Model file for the job. Use its own axes, mm. Face numbers are marked on the shaded views. Give positions to 0.01 mm unless a question says otherwise; leave off trailing zeros. Loops run counter-clockwise (first coordinate to the right, second up) from the corner with the lowest first, then second, coordinate; pieces in that order, holes last. Notation, with made-up numbers: M -13.5,42.5 L 28.5,42.5 A36 ccw 28.5,80.5 Z; hole C 47,-6 d10. An arc over 180 degrees is marked long. Use CSV: the item, a comma, the result in double quotes. Start each with the question number.
(1) Slice it at C-C on x = -41. List the corners of the cut face in (y, z).
(2) Wall check: line 1 along X through (y, z) = (-11, 9); line 2 along X through (y, z) = (10.75, 2.5); line 3 along Y through (x, z) = (-14.5, 2.25). Give the ranges that are in metal, low to high. Write a range as from..to.
(3) Slice it at B-B on y = -5. List the corners of the cut face in (x, z).
(4) Two-plate mould, pull along X, no slides. Class the marked faces 1, 2 and 3: pulls with the +X half, pulls with the -X half, needs draft (parallel to the pull), parting line crosses it, or undercut.
(5) Flat gauge pins, fed straight in: P1, Ø6, axis at x = 19, z = 18.5, coming from the +Y side; P2, Ø5, axis at x = 8.5, z = 11, coming from the +Y side; P3, Ø4, axis at x = 1.5, z = 15.5, coming from the +Y side. Where does each tip first touch, or does it go through?
(6) Slice it at A-A on x = 9. List the corners of the cut face in (y, z), and give its area (3 significant figures).
```python
from build123d import *

# Parameters (mm, degrees)
F0_W     = 101.6
F0_H     = 25.4
F1_DEPTH = 25.4
F3_DEPTH = 101.6
F4_R     = 2.54
F5_R     = 2.667
F6_DEPTH = 4.064
F7_W     = 22.86
F7_H     = 20.81151
F8_DEPTH = 2.54


with BuildPart() as f1:
    # F0 (on Top) → F1 (new body)
    with BuildSketch(Plane.XY):
        with Locations((0, -0.170567)):
            Rectangle(F0_W, F0_H)
    extrude(amount=F1_DEPTH)

    # F2 (on face) → F3 (cut, through all)
    with BuildSketch(Plane(origin=(-50.8, 0, 0), x_dir=(0, -1, 0), z_dir=(-1, 0, 0))):
        Polygon((-12.529433, 25.4), (-12.529433, 8.090758), (-10.742588, 5.36007), (12.870567, 20.81151), (12.870567, 25.4), align=None)
    extrude(amount=-F3_DEPTH, mode=Mode.SUBTRACT)

    # F4
    f4_edges = [f1.edges().sort_by_distance(p)[0] for p in [
        (50.8, 12.529433, 4.045379),
        (50.8, -0.170567, 0),
        (-50.8, -0.170567, 0),
        (-50.8, 12.529433, 4.045379),
        (0, 12.529433, 0),
    ]]
    fillet(f4_edges, radius=F4_R)

    # F5 (on face) → F6 (join)
    with BuildSketch(Plane(origin=(0, 5.676581, 8.675048), x_dir=(1, 0, 0), z_dir=(0, 0.547549, 0.836774))):
        with Locations((-40.64, -3.343786)):
            Circle(F5_R)
    extrude(amount=F6_DEPTH)

    # F7 (on face) → F8 (cut)
    with BuildSketch(Plane.XZ.offset(12.870567)):
        with Locations((6.35, 10.405755)):
            Rectangle(F7_W, F7_H)
    extrude(amount=-F8_DEPTH, mode=Mode.SUBTRACT)


solid = f1.part
```
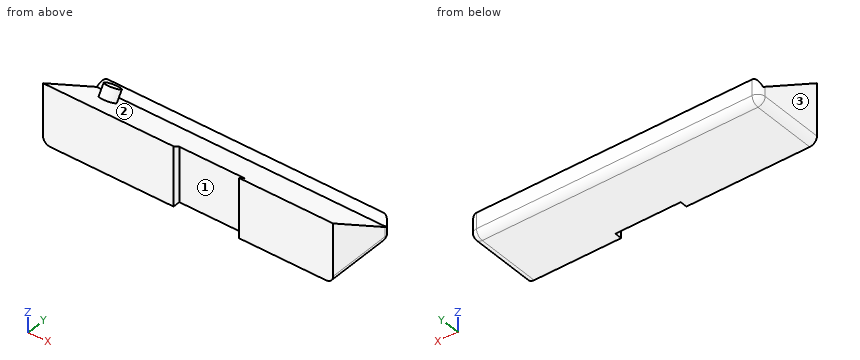
Reply:
1,outline,"M -12.87,0 L 9.99,0 A2.54 ccw 12.53,2.54 L 12.53,8.09 L 10.74,5.36 L 5.09,9.06 L 7.32,12.46 L 2.89,15.35 L 0.67,11.95 L -12.87,20.81 Z"
2,line 1,"x = -50.8..-5.08, 17.78..50.8"
2,line 2,"x = -50.68..50.68"
2,line 3,"y = -12.87..12.51"
3,outline,"M -50.8,2.54 A2.54 ccw -48.26,0 L 48.26,0 A2.54 ccw 50.8,2.54 L 50.8,15.66 L -50.8,15.66 Z"
4,face 1,"undercut"
4,face 2,"needs draft"
4,face 3,"pulls with the -X half"
5,P1,"stops at y = -4.75"
5,P2,"stops at y = 5.94"
5,P3,"stops at y = -1.7"
6,outline,"M -10.33,0 L 9.99,0 A2.54 ccw 12.53,2.54 L 12.53,8.09 L 10.74,5.36 L -10.33,19.15 Z"
6,area,"269 mm^2"
